Work out the finished part from the listing and answer in its coordinate system (mm). Face numbers are marked on the shaded views. A direction names the side the tool comes from. Coordinates: 2 decimals unless noted, no trailing zeros. Order: outer loops, then holes, each group sorted by start corner. A loop starts at its lowest first (then second) coordinate and runs counter-clockwise, first axis right, second up. Notation, with made-up numbers: M 82,79 L 96,79 A28 ccw 96,100 Z; hole C 59.5,73.25 d1. An arc over 180 degrees is marked long. Write item = value, one per line. Start each with the question number.
Q1. Find section C-C on x = 48. Give the vertices of the cut face in (y, z), and give its area (3 significant figures).
Q2. A tool of negligible diameter and unlimited length cuts with its end or side. For the marked faces 1, 2 and 3, from which of +Z, -Z, +X, -X, +Y, -Y can it reach the whole face along a straight path? Write none if from no direction.
Q3. Straight lines are drawn through the part: line 1 along X through (y, z) = (3, -7); line 2 along Z through (x, y) = (64, 30.5); line 3 along X through (y, z) = (8, -43). For each, find the intervals that lie inside material, in ascending order.
Q4. Find section A-A on y = 14. Give the vertices of the cut face in (x, z).
Q5. Find section B-B on z = -45. Give the vertices of the cut face in (x, y).
Q6. Find section D-D on z = -35. Give the vertices of the cut face in (x, y), and give its area (3 significant figures).
Q7. Each of these flat-tipped pins is pushed along its axis until it touches: P1, Ø16.5, axis at x = 53.5, y = 20.5, coming from the -Z side; P2, Ø1, axis at y = 15, z = -38, coming from the -X side; P3, Ø3.5, axis at y = 20.5, z = -44.5, coming from the +X side. Where does it stop, or does it pass through?
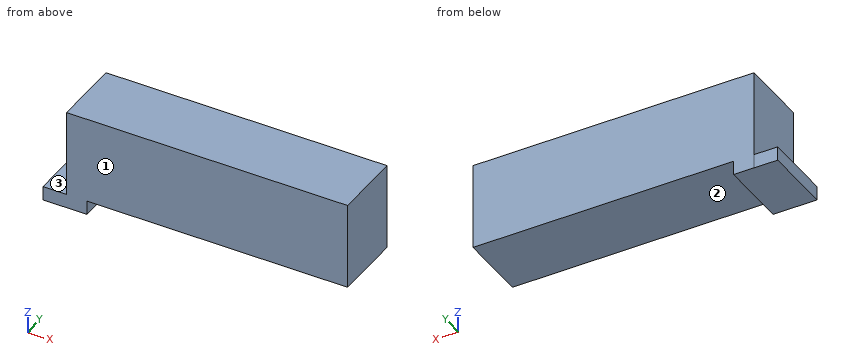
```python
from build123d import *

# Parameters (mm, degrees)
SKETCH2_W           = 135.26
SKETCH2_H           = 41.91
BOSS_EXTRUDE1_DEPTH = 33.16
SKETCH3_W           = 9.84
SKETCH3_H           = 6.82
BOSS_EXTRUDE2_DEPTH = 33.16
SKETCH7_W           = 11.33
SKETCH7_H           = 33.072325858
BOSS_EXTRUDE3_DEPTH = 6.82


with BuildPart() as part:
    # Sketch2 → Boss-Extrude1 (new body)
    with BuildSketch(Plane(origin=(0, 0, 0), x_dir=(1, 0, 0), z_dir=(0, 1, 0))):
        with Locations((67.63, 20.955)):
            Rectangle(SKETCH2_W, SKETCH2_H)
    extrude(amount=BOSS_EXTRUDE1_DEPTH)

    # Sketch3 → Boss-Extrude2 (add)
    with BuildSketch(Plane(origin=(0, 0, 0), x_dir=(1, 0, 0), z_dir=(0, 1, 0))):
        with Locations((4.92, 45.32)):
            Rectangle(SKETCH3_W, SKETCH3_H)
    extrude(amount=BOSS_EXTRUDE2_DEPTH)

    # Sketch7 → Boss-Extrude3 (add)
    with BuildSketch(Plane(origin=(0, 0, -48.73), x_dir=(-1, 0, 0), z_dir=(0, 0, -1))):
        with Locations((5.665, 16.536162929)):
            Rectangle(SKETCH7_W, SKETCH7_H)
    extrude(amount=-BOSS_EXTRUDE3_DEPTH)


solid = part.part
```
Findings below:
q1.outline = M 0,-41.91 L 33.16,-41.91 L 33.16,0 L 0,0 Z
q1.area = 1,390 mm^2
q2.face_1 = +Z, -Z, +X, -X, -Y
q2.face_2 = -Z, +X, +Y, -Y
q2.face_3 = +Z, -X, +Y, -Y
q3.line_1 = 0 to 135.26
q3.line_2 = -41.91 to 0
q3.line_3 = -11.33 to 9.84
q4.outline = M -11.33,-48.73 L 9.84,-48.73 L 9.84,-41.91 L 135.26,-41.91 L 135.26,0 L 0,0 L 0,-41.91 L -11.33,-41.91 Z
q5.outline = M -11.33,0 L 9.84,0 L 9.84,33.16 L 0,33.16 L 0,33.07 L -11.33,33.07 Z
q6.outline = M 0,0 L 135.26,0 L 135.26,33.16 L 0,33.16 Z
q6.area = 4,490 mm^2
q7.P1 = -41.91
q7.P2 = 0
q7.P3 = 9.84
